from build123d import *

# Parameters (mm, degrees)
BOSS_EXTRUDE1_DEPTH = 6.35
CUT_EXTRUDE1_REACH  = 8.35
SKETCH2_W           = 29.21
SKETCH2_H           = 29.21
FILLET1_R           = 5.08
BOSS_EXTRUDE2_DEPTH = 6.35
FILLET2_R           = 2.54


with BuildPart() as part:
    # Sketch1 → Boss-Extrude1 (new body)
    with BuildSketch(Plane.XY):
        with BuildLine():
            ThreePointArc((42.457951031, 57.15), (0, 85.455300688), (-42.457951031, 57.15))
            ThreePointArc((-42.457951031, 57.15), (-48.776790726, 27.667949622), (-44.086837414, -2.116666667))
            ThreePointArc((-44.086837414, -2.116666667), (0, -33.290768363), (44.086837414, -2.116666667))
            ThreePointArc((44.086837414, -2.116666667), (48.776790726, 27.667949622), (42.457951031, 57.15))
        make_face()
        with BuildLine():
            ThreePointArc((-38.1, 0), (-42.411411047, 22.737195516), (-39.698659089, 45.72))
            Line((-39.698659089, 45.72), (39.698659089, 45.72))
            ThreePointArc((39.698659089, 45.72), (42.411411047, 22.737195516), (38.1, 0))
            ThreePointArc((38.1, 0), (0, -26.940768363), (-38.1, 0))
        make_face(mode=Mode.SUBTRACT)
    extrude(amount=BOSS_EXTRUDE1_DEPTH)

    # Sketch2 → Cut-Extrude1 (cut, up to next)
    with BuildSketch(Plane.XY.offset(6.35), mode=Mode.PRIVATE) as cut_extrude1_sk1:
        with Locations((0, 64.135)):
            Rectangle(SKETCH2_W, SKETCH2_H)
    cut_extrude1_tool1 = extrude(cut_extrude1_sk1.sketch, amount=-CUT_EXTRUDE1_REACH, mode=Mode.PRIVATE) & part.part
    add(cut_extrude1_tool1.solids().sort_by_distance((0, 64.135, 6.35))[0], mode=Mode.SUBTRACT)

    # Fillet1
    fillet1_edges = [part.edges().sort_by_distance(p)[0] for p in [
        (14.605, 78.74, 3.175),
        (14.605, 49.53, 3.175),
        (-14.605, 49.53, 3.175),
        (-14.605, 78.74, 3.175),
    ]]
    fillet(fillet1_edges, radius=FILLET1_R)

    # Sketch3 → Boss-Extrude2 (add)
    with BuildSketch(Plane.XY.offset(6.35)):
        Polygon((-38.423965284, 47.135690893), (-40.973352894, 44.304309107), (-2.846977827, 9.975166803), (-31.416785414, -15.749203493), (-28.867397804, -18.580585278), (0, 7.411736453), (28.867397804, -18.580585278), (31.416785414, -15.749203493), (2.846977827, 9.975166803), (40.973352894, 44.304309107), (38.423965284, 47.135690893), (0, 12.538597153), align=None)
    extrude(amount=-BOSS_EXTRUDE2_DEPTH)

    # Fillet2
    fillet2_edges = [part.edges().sort_by_distance(p)[0] for p in [
        (-2.846977827, 9.975166803, 3.175),
        (2.846977827, 9.975166803, 3.175),
        (-40.241399563, 43.645255368, 3.175),
        (29.56358846, -14.08057746, 3.175),
        (26.831630213, -16.747571906, 3.175),
        (-36.851681262, 45.72, 3.175),
        (40.241399563, 43.645255368, 3.175),
        (36.851681262, 45.72, 3.175),
        (0, 12.538597153, 3.175),
        (-29.56358846, -14.08057746, 3.175),
        (-26.831630213, -16.747571906, 3.175),
        (0, 7.411736453, 3.175),
    ]]
    fillet(fillet2_edges, radius=FILLET2_R)


solid = part.part
The listing builds one solid part. Answer for the finished solid, in the listing's coordinates (mm). Round coordinates to 2 decimals unless told otherwise and drop trailing zeros. Write each loop counter-clockwise with the first axis right and the second up, starting at its lowest first coordinate (ties: lowest second). Pieces come first, ordered by that corner, then holes. Notation, with made-up numbers: (86.5, 11.25) - (132.5, 11.25) arc R9 ccw to (132.5, 22.25) - close; hole circle Ø4 at (48.5, -11.5). An arc over 180 degrees is marked (long way). Use a Markdown table: item, result. Add a question column.
1. Consider line 1 (X direction, y = -2, z = 4.5); line 2 (Y direction, x = -22.5, z = 4.25); line 3 (X direction, y = 29.5, z = 3.5). Determine where each line is inside the solid, lowest interval first.
2. The part is cut by section C-C (y = 16.5). Write down the section's boundary in (x, z), and give its area (3 significant figures).
3. The part is cut by section D-D (z = 4.75). Give the number of separate pieces and of enclosed holes in the cut face, and give its area (3 significant figures).
4. Flat-ended cylindrical pins translate along their axes: P1, Ø3, axis at y = 68.5, z = 2.5, coming from the +X side; P2, Ø3, axis at x = -2, z = 4, coming from the -Y side; P3, Ø2, axis at x = -23, z = 3.5, coming from the -Y side. Find the tip coordinate at first contact, or state that the pin passes through.
5. The part is cut by section B-B (x = 22). Write down the section's boundary in (y, z), and give its area (3 significant figures).
6. For a pull along X with two mould halves and no side action, classify faces 1 (the face through (39.465, 41.242, 3.131)), 2 (the face through (0.026, 6.534, 3.131)), 3 (the face through (-48.764, 28.092, 3.131)), 4 (the face through (21, 27, 6.35)) as +X half, -X half, draft (parallel to the pull), parting line (faces both ways), or undercut.
7. The part is cut by section A-A (y = 65). Write down the section's boundary in (x, z) (3 decimals).
Reported:
| question | item | result |
|---|---|---|
| 1 | line 1 | -44.13 to -37.33, -16.15 to -10.45, 10.45 to 16.15, 37.33 to 44.13 |
| 1 | line 2 | -27.52 to -20.1, -12.85 to -7.72, 27.67 to 32.8, 45.72 to 79.58 |
| 1 | line 3 | -48.71 to -42.35, -24.53 to -18.84, 18.84 to 24.53, 42.35 to 48.71 |
| 2 | outline | (-48.33, 0) - (-41.94, 0) - (-41.94, 6.35) - (-48.33, 6.35) - close; (-10.09, 0) - (-4.4, 0) - (-4.4, 6.35) - (-10.09, 6.35) - close; (4.4, 0) - (10.09, 0) - (10.09, 6.35) - (4.4, 6.35) - close; (41.94, 0) - (48.33, 0) - (48.33, 6.35) - (41.94, 6.35) - close |
| 2 | area | 153 mm^2 |
| 3 | separate pieces | 1 |
| 3 | enclosed holes | 5 |
| 3 | area | 3,920 mm^2 |
| 4 | P1 | x = 36.84 |
| 4 | P2 | y = -33.29 |
| 4 | P3 | y = -27.79 |
| 5 | outline | (-27.79, 0) - (-20.43, 0) - (-20.43, 6.35) - (-27.79, 6.35) - close; (-12.4, 0) - (-7.27, 0) - (-7.27, 6.35) - (-12.4, 6.35) - close; (27.22, 0) - (32.35, 0) - (32.35, 6.35) - (27.22, 6.35) - close; (45.72, 0) - (79.85, 0) - (79.85, 6.35) - (45.72, 6.35) - close |
| 5 | area | 329 mm^2 |
| 6 | face 1 | undercut |
| 6 | face 2 | undercut |
| 6 | face 3 | -X half |
| 6 | face 4 | draft |
| 7 | outline | (-38.253, 0) - (-14.605, 0) - (-14.605, 6.35) - (-38.253, 6.35) - close; (14.605, 0) - (38.253, 0) - (38.253, 6.35) - (14.605, 6.35) - close |
